from build123d import *

# Parameters (mm, degrees)
SKETCH1_R               = 5.08
SKETCH1_R_2             = 1.5875
BOSS_EXTRUDE1_DEPTH     = 3.81
SKETCH2_R               = 2.54
SKETCH2_R_2             = 1.5875
BOSS_EXTRUDE2_DEPTH     = 3.175
SKETCH3_R               = 4.7625
SKETCH3_R_2             = 1.5875
BOSS_EXTRUDE3_DEPTH     = 3.81
CHAMFER1_SIZE           = 0.508
CHAMFER2_SIZE           = 0.508
CHAMFER3_SIZE           = 2.032
CUT_EXTRUDE1_DEPTH      = 13.967066939
CUT_EXTRUDE1_DEPTH_BACK = 13.967066939
SKETCH4_R               = 40.64
CHAMFER4_SIZE           = 1.016


with BuildPart() as part:
    # Sketch1 → Boss-Extrude1 (new body)
    with BuildSketch(Plane.XY):
        with Locations(Location((0, 0, 0), (0, 0, 180))):
            Circle(SKETCH1_R)
        with Locations(Location((0, 0, 0), (0, 0, 180))):
            Circle(SKETCH1_R_2, mode=Mode.SUBTRACT)
    extrude(amount=BOSS_EXTRUDE1_DEPTH)

    # Sketch2 → Boss-Extrude2 (add)
    with BuildSketch(Plane.XY.offset(3.81)):
        Circle(SKETCH2_R)
        with Locations(Location((0, 0, 0), (0, 0, 180))):
            Circle(SKETCH2_R_2, mode=Mode.SUBTRACT)
    extrude(amount=BOSS_EXTRUDE2_DEPTH)

    # Sketch3 → Boss-Extrude3 (add)
    with BuildSketch(Plane.XY.offset(6.985)):
        with Locations(Location((0, 0, 0), (0, 0, 180))):
            Circle(SKETCH3_R)
        with Locations(Location((0, 0, 0), (0, 0, 180))):
            Circle(SKETCH3_R_2, mode=Mode.SUBTRACT)
    extrude(amount=BOSS_EXTRUDE3_DEPTH)

    # Chamfer1
    chamfer1_edges = [part.edges().sort_by_distance(p)[0] for p in [
        (-2.54, 0, 6.985),
        (-2.54, 0, 3.81),
    ]]
    chamfer(chamfer1_edges, length=CHAMFER1_SIZE)

    # Chamfer2
    chamfer2_edges = [part.edges().sort_by_distance(p)[0] for p in [
        (4.7625, 0, 6.985),
        (5.08, 0, 3.81),
    ]]
    chamfer(chamfer2_edges, length=CHAMFER2_SIZE)

    # Chamfer3
    chamfer3_edges = [part.edges().sort_by_distance(p)[0] for p in [
        (1.5875, 0, 10.795),
    ]]
    chamfer(chamfer3_edges, length=CHAMFER3_SIZE)

    # Sketch4 → Cut-Extrude1 (cut, two sides: drawn at the far end of the back side and taken through both)
    with BuildSketch(Plane(origin=(0, 0, 0), x_dir=(0, 0, -1), z_dir=(1, 0, 0)).offset(-CUT_EXTRUDE1_DEPTH_BACK)):
        with Locations((40.321249981, 0)):
            Circle(SKETCH4_R)
    extrude(amount=CUT_EXTRUDE1_DEPTH + CUT_EXTRUDE1_DEPTH_BACK, mode=Mode.SUBTRACT)

    # Chamfer4
    chamfer4_edges = [part.edges().sort_by_distance(p)[0] for p in [
        (4.7625, 0, 10.795),
    ]]
    chamfer(chamfer4_edges, length=CHAMFER4_SIZE)


solid = part.part
For this review, take the finished solid that the model builds, in its own axes (mm). A direction names the side the tool comes from. Give positions to 0.01 mm unless a question says otherwise; leave off trailing zeros. Order: outer loops, then holes, each group sorted by start corner. A loop starts at its lowest first (then second) coordinate and runs counter-clockwise, first axis right, second up. Notation, with made-up numbers: (40, 21) - (84, 21) arc R19 cw to (84, 56) - close; hole circle Ø7 at (82, 35.5). An arc over 180 degrees is marked (long way). Answer as a JSON object with one key per item and string values. Group by question number.
Item 1: Clearance check with flat-ended pins moving along their axes: pin 1 Ø1.5 at (y, z) = (2, 8) entering from +X; pin 2 Ø1.5 at (y, z) = (1, 7.5) entering from -X; pin 3 Ø4.5 at (x, y) = (0.5, 0.5) entering from -Z; pin 4 Ø5 at (x, z) = (1.5, 4) entering from +Y. State where each tip first meets the part, or that it passes through.
Item 2: Take a section at C-C on z = 5. Give the boundary of the cut face in (x, y) (1 decimal).
Item 3: Draft analysis for pull direction Y (two halves, no side actions). For faces 1 (the cylindrical face through (1.03, 4.65, 8.62)), 2 (the flat face through (-2, 3, 6.985)), 3 (the conical face through (-0.79, 1.52, 8.89)), state which applies: pulls with the +Y half, pulls with the -Y half, needs draft (parallel to the pull), parting line crosses it, or undercut.
Item 4: Machinability: for faces 4 (the cylindrical face through (-1.514, -0.477, 4.466)), 5 (the cylindrical face through (-0.33, 2.52, 5.38)), which of the approach directions +Z, -Z, +X, -X, +Y, -Y give a long, thin tool a straight path to every point of the face, cutting with its end or side? Answer none if there is none.
Item 5: Wall thickness on line 1 along Y through (x, z) = (0, 6); line 2 along Y through (x, z) = (0, 2.75); line 3 along Z through (x, y) = (3.75, 1) (3 decimals): over which ranges is each line inside the solid? List them lowest first.
Reported:
{
 "1": {"pin 1": "x = 4.6", "pin 2": "x = -4.76", "pin 3": "z = 0.23", "pin 4": "y = 5.08"},
 "2": {"outline": "circle Ø5.1 at (0, 0); hole circle Ø3.2 at (0, 0)"},
 "3": {"face 1": "parting line crosses it", "face 2": "needs draft", "face 3": "undercut"},
 "4": {"face 4": "+Z, -Z", "face 5": "none"},
 "5": {"line 1": "-2.54 to -1.59, 1.59 to 2.54", "line 2": "-5.08 to -1.59, 1.59 to 5.08", "line 3": "0.306 to 3.81, 6.985 to 10.66"}
}
